Part model, mm, in its own coordinate system. A direction names the side the tool comes from. Give positions to 0.01 mm unless a question says otherwise; leave off trailing zeros. Order: outer loops, then holes, each group sorted by start corner. A loop starts at its lowest first (then second) coordinate and runs counter-clockwise, first axis right, second up. Notation, with made-up numbers: M 51.5,38 L 69.5,38 A11 ccw 69.5,44 Z; hole C 27.5,-3 d8. An arc over 180 degrees is marked long. Return JSON: item names as keys, results as strings.
from build123d import *

# Parameters (mm, degrees)
SKETCH1_R           = 12.5
BOSS_EXTRUDE1_DEPTH = 650
SKETCH3_R           = 11
BOSS_EXTRUDE2_DEPTH = 70


with BuildPart() as part:
    # Sketch1 → Boss-Extrude1 (new body)
    with BuildSketch(Plane.XY):
        Circle(SKETCH1_R)
    extrude(amount=BOSS_EXTRUDE1_DEPTH)

    # Sketch2 → Revolve1 (revolve)
    with BuildSketch(Plane(origin=(0, 0, 0), x_dir=(1, 0, 0), z_dir=(0, 1, 0)), mode=Mode.PRIVATE) as revolve1_sk:
        Polygon((0, -650), (0, -662.5), (12.5, -650), align=None)
    revolve(revolve1_sk.sketch.rotate(Axis((0, 0, 650), (0, 0, 1)), 180), axis=Axis((0, 0, 650), (0, 0, 1)))

    # Sketch3 → Boss-Extrude2 (add)
    with BuildSketch(Plane(origin=(0, 0, 0), x_dir=(-1, 0, 0), z_dir=(0, 0, -1))):
        Circle(SKETCH3_R)
    extrude(amount=BOSS_EXTRUDE2_DEPTH)


solid = part.part
Q1. Pin check, flat tips, straight feed: pin 1 (10 mm diameter, centred on x = -5, z = 37.5, fed in from -Y); pin 2 (1.5 mm diameter, centred on y = -4.5, z = 165, fed in from +X); pin 3 (1.5 mm diameter, centred on y = 9.5, z = 76.5, fed in from -X); pin 4 (1 mm diameter, centred on x = 9, y = -0.5, fed in from +Z). Stop position of each tip, or through.
Established:
{"pin 1": "stops at y = -12.5", "pin 2": "stops at x = 11.92", "pin 3": "stops at x = -8.93", "pin 4": "stops at z = 653.99"}
Q2. Band-saw the part on A-A (z = 204). Give the cut face in (x, y), then the cut area to 3 significant figures.
Established:
{"outline": "C 0,0 d25", "area": "491 mm²"}
Q3. 3-axis set-ups, long thin cutter, end or side, ignore diameter. For faces 1 (the cylindrical face through (2.38, -10.74, -34.51)), 2 (the conical face through (-1.914, -3.002, 658.94)): which of +Z, -Z, +X, -X, +Y, -Y reach the whole face in a straight line?
Established:
{"face 1": "-Z", "face 2": "+Z"}
Q4. Probe line 1 along Y through (x, z) = (-1, 192.5); line 2 along X through (y, z) = (-0.5, 218); line 3 along Y through (x, z) = (-6, 583). List the from-to ranges inside material, lowest first.
Established:
{"line 1": "y = -12.46 to 12.46", "line 2": "x = -12.49 to 12.49", "line 3": "y = -10.97 to 10.97"}
